Here's how the part is built. I have some questions about the finished solid (model axes, mm). Face numbers are marked on the shaded views. Give positions to 0.01 mm unless a question says otherwise; leave off trailing zeros. Loops run counter-clockwise (first coordinate to the right, second up) from the corner with the lowest first, then second, coordinate; pieces in that order, holes last.
Q1. Will these pins go through, and if not, where does the flat tip stop? P1, Ø5, axis at x = -1, y = 1.5, coming from the -Z side; P2, Ø8, axis at x = 4.5, y = 5.5, coming from the +Z side.
Q2. I need wall thicknesses on line 1 (Y direction, x = -0.5, z = -0.35); line 2 (Y direction, x = 0, z = -0.75); line 3 (X direction, y = 2.5, z = -1.2). Which ranges of each line are inside material? Lowest first, please.
Q3. We'd pull the mould along Y, two halves only. Please class the marked faces 1 and 2: +Y half, -Y half, draft (parallel to the pull), parting line (faces both ways), or undercut.
Q4. If we section it at D-D (z = -1.5): Please give me the cut outline in (x, y), plus the area to 3 significant figures.
Q5. If we section it at C-C (z = -0.4): Please give me the cut outline in (x, y), plus the area to 3 significant figures.
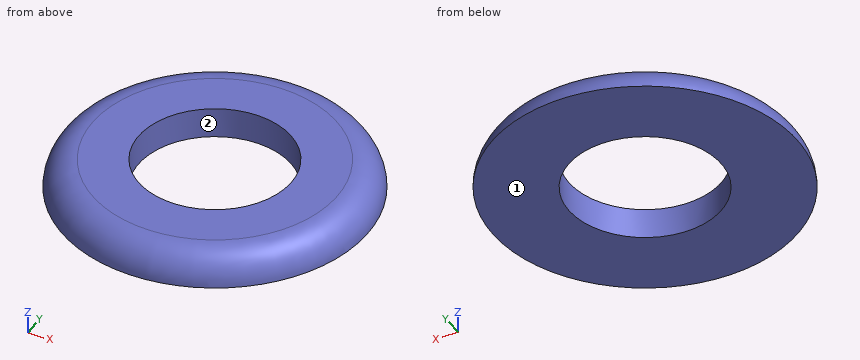
from build123d import *

# Parameters (mm, degrees)
F0_R     = 10
F1_DEPTH = 2
F2_R     = 1.99999
F3_R     = 5
F4_DEPTH = 25


# Not quite as in the source:
# - a fillet or chamfer is up to 0.001 mm smaller than in the source, because OpenCascade refuses the exact size


with BuildPart() as f1:
    # F0 (on Top) → F1 (new body)
    with BuildSketch(Plane.XY):
        Circle(F0_R)
    extrude(amount=-F1_DEPTH)

    # F2 (radius 2 in the source; OpenCascade refuses exactly that, so slightly less here)
    f2_edges = [f1.edges().sort_by_distance(p)[0] for p in [
        (-10, 0, 0),
    ]]
    fillet(f2_edges, radius=F2_R)

    # F3 (on face) → F4 (cut)
    with BuildSketch(Plane.XY):
        Circle(F3_R)
    extrude(amount=-F4_DEPTH, mode=Mode.SUBTRACT)


solid = f1.part
Check sheet entries:
1. P1: passes through
1. P2: stops at z = 0
2. line 1: y = -9.12 to -4.97, 4.97 to 9.12
2. line 2: y = -9.56 to -5, 5 to 9.56
2. line 3: x = -9.51 to -4.33, 4.33 to 9.51
3. face 1: draft
3. face 2: undercut
4. outline: circle Ø19.87 at (0, 0); hole circle Ø10 at (0, 0)
4. area: 232 mm2
5. outline: circle Ø18.4 at (0, 0); hole circle Ø10 at (0, 0)
5. area: 187 mm2
